Check sheet for the drawn part. Datum: minimum x, y, z corner. Units: mm. A direction names the side the tool comes from. Give positions to 0.01 mm unless a question says otherwise; leave off trailing zeros. Write each loop counter-clockwise with the first axis right and the second up, starting at its lowest first coordinate (ties: lowest second). Pieces come first, ordered by that corner, then holes.
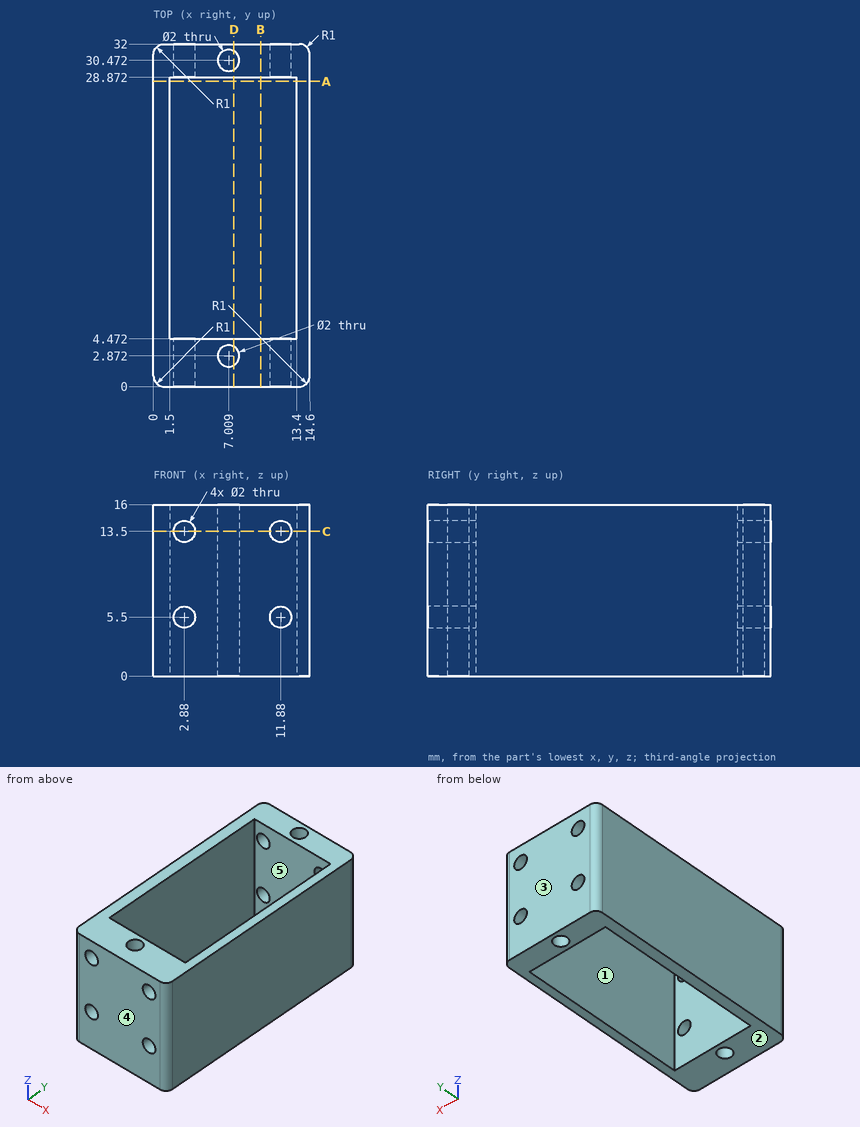
1) Scan lines: L1, parallel to X at y = 2.75, z = 5.5; L2, parallel to Y at x = 5.25, z = 4.5; L3, parallel to X at y = 5.5, z = 12.5. Record each from-to range of solid material in increasing order.
2) Sectioned sample at B-B on x = 10. Record the boundary of the cut face in (y, z), then the cut area to 3 significant figures.
3) Sectioned sample at C-C on z = 13.5. Give the number of separate pieces and of enclosed holes in the cut face, then the cut area to 3 significant figures.
4) Draft check along Y on the marked faces 3, 4 and 5. Enter one of: +Y half, -Y half, draft (parallel to the pull), parting line (faces both ways), or undercut.
5) Access from +Z, -Z, +X, -X, +Y, -Y to the whole of each face (thin tool, end or side, straight path). Record for the marked faces 1 and 2.
6) Sectioned sample at A-A on y = 28.5. Record the boundary of the cut face in (x, z).
7) Sectioned sample at D-D on x = 7.5. Record the boundary of the cut face in (y, z).
8) Gauge pin test, flat ends, axial feed: pin 1 (3 mm diameter, centred on x = 11.5, y = 10.5, fed in from +Z); pin 2 (2.5 mm diameter, centred on x = 11.88, z = 5.5, fed in from -Y). Record the tip position at first contact, or that the pin passes through.
Answers below:
1. L1: x = 0 to 1.88, 3.88 to 6.02, 8 to 10.88, 12.88 to 14.6
1. L2: y = 0 to 4.47, 28.87 to 32
1. L3: x = 0 to 1.5, 13.4 to 14.6
2. outline: (0, 0) - (4.47, 0) - (4.47, 16) - (0, 16) - close; (28.87, 0) - (32, 0) - (32, 16) - (28.87, 16) - close
2. area: 122 mm2
3. separate pieces: 4
3. enclosed holes: 2
3. area: 139 mm2
4. face 3: +Y half
4. face 4: -Y half
4. face 5: undercut
5. face 1: +Z, -Z
5. face 2: -Z, +X, -X, +Y, -Y
6. outline: (0, 0) - (1.5, 0) - (1.5, 16) - (0, 16) - close; (13.4, 0) - (14.6, 0) - (14.6, 16) - (13.4, 16) - close
7. outline: (0, 0) - (2, 0) - (2, 16) - (0, 16) - close; (3.74, 0) - (4.47, 0) - (4.47, 16) - (3.74, 16) - close; (28.87, 0) - (29.6, 0) - (29.6, 16) - (28.87, 16) - close; (31.34, 0) - (32, 0) - (32, 16) - (31.34, 16) - close
8. pin 1: passes through
8. pin 2: stops at y = 0
